from build123d import *

# Parameters (mm, degrees)
SKETCH1_R           = 2
SKETCH1_R_2         = 2.099997394
SKETCH1_R_3         = 2.100000418
BOSS_EXTRUDE1_DEPTH = 3


with BuildPart() as part:
    # Sketch1 → Boss-Extrude1 (new body)
    with BuildSketch(Plane.XY):
        with BuildLine():
            Line((243.514566495, 346.287321237), (313.514566495, 346.287321237))
            ThreePointArc((313.514566495, 346.287321237), (348.514566495, 311.287321237), (313.514566495, 276.287321237))
            Line((313.514566495, 276.287321237), (243.514566495, 276.287321237))
            ThreePointArc((243.514566495, 276.287321237), (208.514566495, 311.287321237), (243.514566495, 346.287321237))
        make_face()
        with Locations((243.514566495, 311.287321237)):
            Circle(SKETCH1_R, mode=Mode.SUBTRACT)
        with Locations((313.514566495, 311.287321237)):
            Circle(SKETCH1_R, mode=Mode.SUBTRACT)
        with Locations((246.764562225, 324.225588056)):
            Circle(SKETCH1_R_2, mode=Mode.SUBTRACT)
        with Locations((229.564568056, 323.725595013)):
            Circle(SKETCH1_R_3, mode=Mode.SUBTRACT)
        with Locations((278.514566495, 342.287321237)):
            Circle(SKETCH1_R, mode=Mode.SUBTRACT)
        with Locations(Location((278.514566495, 280.287321237, 0), (0, 0, 180))):
            Circle(SKETCH1_R, mode=Mode.SUBTRACT)
    extrude(amount=BOSS_EXTRUDE1_DEPTH)


solid = part.part
Work out the finished part from the listing and answer in its coordinate system (mm). Give positions to 0.01 mm unless a question says otherwise; leave off trailing zeros. Write each loop counter-clockwise with the first axis right and the second up, starting at its lowest first coordinate (ties: lowest second). Pieces come first, ordered by that corner, then holes. Notation, with made-up numbers: (42, 39) - (70, 39) arc R6 ccw to (70, 45) - close; hole circle Ø6 at (-19, 25). An arc over 180 degrees is marked (long way). One line per item, written item: value. Start each with the question number.
1. Find section A-A (z = 0.8). Write down the section's boundary in (x, y).
2. Given pin 1 (5 mm diameter, centred on x = 278.51, y = 342.29, fed in from -Z); pin 2 (3.5 mm diameter, centred on x = 243.51, y = 311.29, fed in from -Z); pin 3 (1.5 mm diameter, centred on y = 285, z = 1, fed in from -X), each flat-ended and moving along its own axis, determine where each tip first touches the part or whether it passes through.
3. Consider probe 1 along X at (y, z) = (311, 1.25); probe 2 along Y at (x, z) = (246, 1.25); probe 3 along X at (y, z) = (341.5, 1.4). Determine where each line is inside the solid, lowest interval first.
4. Find section C-C (x = 219.5). Write down the section's boundary in (y, z).
5. For a pull along X with two mould halves and no side action, classify faces 1 (the cylindrical face through (241.517, 311.375, 1.479)), 2 (the cylindrical face through (208.523, 310.518, 1.479)), 3 (the flat face through (279, 276.287, 1)) as +X half, -X half, draft (parallel to the pull), parting line (faces both ways), or undercut.
6. Find section B-B (y = 292.5). Write down the section's boundary in (x, z).
Geometry results:
1. outline: (243.51, 276.29) - (313.51, 276.29) arc R35 ccw to (313.51, 346.29) - (243.51, 346.29) arc R35 ccw to start; hole circle Ø4.2 at (229.56, 323.73); hole circle Ø4 at (243.51, 311.29); hole circle Ø4.2 at (246.76, 324.23); hole circle Ø4 at (278.51, 280.29); hole circle Ø4 at (278.51, 342.29); hole circle Ø4 at (313.51, 311.29)
2. pin 1: z = 0
2. pin 2: through
2. pin 3: x = 219.58
3. probe 1: 208.52 to 241.54, 245.49 to 311.54, 315.49 to 348.51
3. probe 2: 276.29 to 322.27, 326.18 to 346.29
3. probe 3: 225.85 to 276.68, 280.35 to 331.18
4. outline: (285.83, 0) - (336.75, 0) - (336.75, 3) - (285.83, 3) - close
5. face 1: undercut
5. face 2: -X half
5. face 3: draft
6. outline: (213.98, 0) - (343.04, 0) - (343.04, 3) - (213.98, 3) - close
